For this review, take the finished solid that the model builds, in its own axes (mm). A direction names the side the tool comes from. Give positions to 0.01 mm unless a question says otherwise; leave off trailing zeros. Order: outer loops, then holes, each group sorted by start corner. A loop starts at its lowest first (then second) coordinate and runs counter-clockwise, first axis right, second up. Notation, with made-up numbers: M 71.25,-16.75 L 116.25,-16.75 A28 ccw 116.25,9.25 Z; hole C 20.25,-24 d9. An arc over 180 degrees is marked long. Answer as CSV lines item,"result". Start each with the question number.
1. We need section D-D, the plane z = -9.5. Give the boundary of the cut face in (x, y).
2. Mouldability with a two-part tool opening along X and no side actions: class faces 1 (the flat face through (-13, 4.8, -32)), 2 (the flat face through (-3.35, 20, -1)) as pulls with the +X half, pulls with the -X half, needs draft (parallel to the pull), parting line crosses it, or undercut.
3. We need section A-A, the plane y = 18. Give the boundary of the cut face in (x, z), and give its area (3 significant figures).
4. We need section B-B, the plane z = -16. Give the boundary of the cut face in (x, y), and give its area (3 significant figures).
5. For line 1 along X through (y, z) = (12.5, -6.5); line 2 along Y through (x, z) = (10.25, -8.5); line 3 along Z through (x, y) = (-2, 29.5), list the stretches that pass through material, from the lowest coordinate up.
6. Clearance check with flat-ended pins moving along their axes: P1, Ø11, axis at x = 2, z = -18.5, coming from the +Y side; P2, Ø3, axis at x = -12, y = 32.5, coming from the -Z side; P3, Ø1.4, axis at x = 13.5, z = -31.5, coming from the +Y side. State where each tip first meets the part, or that it passes through.
7. Machinability: for faces 3 (the cylindrical face through (-0.07, 12.15, -1.42)), 4 (the flat face through (3.35, 1, -20)), 5 (the flat face through (3, 0, -13)), 6 (the flat face through (-11.2, 12, -12)), 7 (the flat face through (13, 4.8, -32)), which of the approach directions +Z, -Z, +X, -X, +Y, -Y give a long, thin tool a straight path to every point of the face, cutting with its end or side? Answer none if there is none.
8. We need section C-C, the plane x = 2. Give the boundary of the cut face in (y, z), and give its area (3 significant figures).
from build123d import *

# Parameters (mm, degrees)
EXTRUDE_1_DEPTH     = 14
EXTRUDE_3_DEPTH     = 2.8
FILLET_1_R          = 1
CUT_EXTRUDE_1_DEPTH = 2.8
CUT_EXTRUDE_2_DEPTH = 2.8


with BuildPart() as part:
    # 草图1 → 凸台-拉伸1 (new body, symmetric)
    with BuildSketch(Plane(origin=(0, 0, 0), x_dir=(0, 0, -1), z_dir=(1, 0, 0))):
        Polygon((0, 34.8), (0, 0), (34.8, 0), (34.8, 2.8), (2.8, 2.8), (2.8, 34.8), align=None)
    extrude(amount=EXTRUDE_1_DEPTH, both=True)

    # 草图2 → 凸台-拉伸3 (add)
    with BuildSketch(Plane(origin=(14, 0, 0), x_dir=(0, 0, -1), z_dir=(1, 0, 0))):
        Polygon((2.8, 34.8), (4.8, 34.8), (4.8, 29.8), (29.8, 4.8), (34.8, 4.8), (34.8, 2.8), (2.8, 2.8), align=None)
    extrude_3 = extrude(amount=-EXTRUDE_3_DEPTH)

    # 镜向1: 凸台-拉伸3 across plane
    add(extrude_3.mirror(Plane(origin=(0, 0, 0), x_dir=(0, 0, 1), z_dir=(1, 0, 0))))

    # 圆角1
    fillet_1_edges = [part.edges().sort_by_distance(p)[0] for p in [
        (12.6, 34.8, -4.8),
        (12.6, 29.8, -4.8),
        (12.6, 4.8, -29.8),
        (12.6, 4.8, -34.8),
        (-12.6, 4.8, -34.8),
        (-12.6, 4.8, -29.8),
        (-12.6, 29.8, -4.8),
        (-12.6, 34.8, -4.8),
    ]]
    fillet(fillet_1_edges, radius=FILLET_1_R)

    # 草图3 → 切除-拉伸1 (cut)
    with BuildSketch(Plane(origin=(0, 2.8, 0), x_dir=(1, 0, 0), z_dir=(0, 1, 0))):
        with BuildLine():
            Line((-3.35, 15.5), (-3.35, 24.1))
            ThreePointArc((-3.35, 24.1), (0, 27.45), (3.35, 24.1))
            Line((3.35, 24.1), (3.35, 15.5))
            ThreePointArc((3.35, 15.5), (0, 12.15), (-3.35, 15.5))
        make_face()
    extrude(amount=-CUT_EXTRUDE_1_DEPTH, mode=Mode.SUBTRACT)

    # 草图4 → 切除-拉伸2 (cut)
    with BuildSketch(Plane(origin=(0, 0, -2.8), x_dir=(-1, 0, 0), z_dir=(0, 0, -1))):
        with BuildLine():
            Line((-3.35, 15.5), (-3.35, 24.1))
            ThreePointArc((-3.35, 24.1), (0, 27.45), (3.35, 24.1))
            Line((3.35, 24.1), (3.35, 15.5))
            ThreePointArc((3.35, 15.5), (0, 12.15), (-3.35, 15.5))
        make_face()
    extrude(amount=-CUT_EXTRUDE_2_DEPTH, mode=Mode.SUBTRACT)


solid = part.part
Result set:
1,outline,"M -14,0 L 14,0 L 14,25.1 L 11.2,25.1 L 11.2,2.8 L -11.2,2.8 L -11.2,25.1 L -14,25.1 Z"
2,face 1,"needs draft"
2,face 2,"undercut"
3,outline,"M -14,-16.6 L -11.2,-16.6 L -11.2,-2.8 L -3.35,-2.8 L -3.35,0 L -14,0 Z; M 3.35,-2.8 L 11.2,-2.8 L 11.2,-16.6 L 14,-16.6 L 14,0 L 3.35,0 Z"
3,area,"137 mm2"
4,outline,"M -14,0 L -3.35,0 L -3.35,2.8 L -11.2,2.8 L -11.2,18.6 L -14,18.6 Z; M 3.35,0 L 14,0 L 14,18.6 L 11.2,18.6 L 11.2,2.8 L 3.35,2.8 Z"
4,area,"148 mm2"
5,line 1,"-14 to -11.2, 11.2 to 14"
5,line 2,"0 to 2.8"
5,line 3,"-2.8 to 0"
6,P1,"y = 2.8"
6,P2,"z = -4.8"
6,P3,"y = 4.8"
7,face 3,"+Z, -Z"
7,face 4,"+Y, -Y"
7,face 5,"+Z, -Z, +X, -X, -Y"
7,face 6,"-Z, +Y"
7,face 7,"-Z, +X, -X, +Y"
8,outline,"M 0,-34.8 L 2.8,-34.8 L 2.8,-26.79 L 0,-26.79 Z; M 0,-12.81 L 2.8,-12.81 L 2.8,-2.8 L 12.81,-2.8 L 12.81,0 L 0,0 Z; M 26.79,-2.8 L 34.8,-2.8 L 34.8,0 L 26.79,0 Z"
8,area,"109 mm2"
